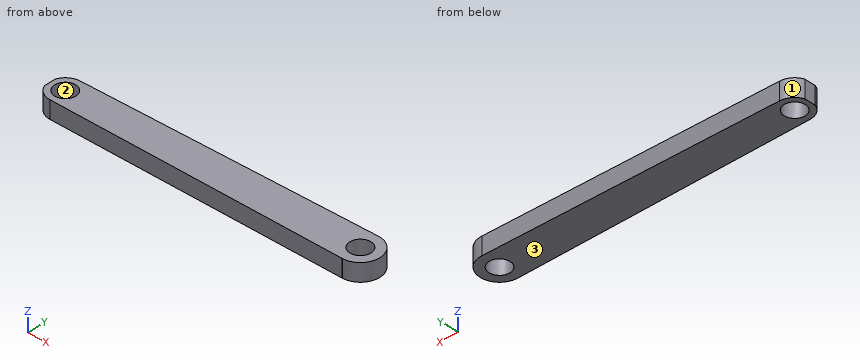
from build123d import *

# Parameters (mm, degrees)
SZKIC1_R                    = 4.635188213
SZKIC1_R_2                  = 3.000000079
SZKIC1_R_3                  = 5.522620658
DODANIE_WYCI_GNI_CIE1_DEPTH = 5
SZKIC2_W                    = 1.618528634
SZKIC2_H                    = 7.505645785
SZKIC2_W_2                  = 0.651830256
SZKIC2_H_2                  = 5.051684483
WYTNIJ_WYCI_GNI_CIE3_DEPTH  = 6


with BuildPart() as part:
    # Szkic1 → Dodanie-wyciągnięcie1 (new body)
    with BuildSketch(Plane.XY):
        with BuildLine():
            Line((0, -4.635188213), (83.645408354, -5.521381009))
            ThreePointArc((83.645408354, -5.521381009), (78.239794892, 0), (83.645408354, 5.521381009))
            Line((83.645408354, 5.521381009), (0, 4.635188213))
            ThreePointArc((0, 4.635188213), (3.277573017, 3.277573017), (4.635188213, 0))
            ThreePointArc((4.635188213, 0), (3.277573017, -3.277573017), (0, -4.635188213))
        make_face()
        Circle(SZKIC1_R)
        Circle(SZKIC1_R_2, mode=Mode.SUBTRACT)
        with BuildLine():
            ThreePointArc((0, 4.635188213), (-4.635188213, 0), (0, -4.635188213))
            ThreePointArc((0, -4.635188213), (3.277573017, -3.277573017), (4.635188213, 0))
            ThreePointArc((4.635188213, 0), (3.277573017, 3.277573017), (0, 4.635188213))
        make_face()
        Circle(SZKIC1_R_2, mode=Mode.SUBTRACT)
        with BuildLine():
            ThreePointArc((83.645408354, -5.521381009), (83.703908669, -5.522310737), (83.76241555, -5.522620658))
            Line((83.76241555, -5.522620658), (83.645408354, -5.521381009))
        make_face()
        with Locations((83.76241555, 0)):
            Circle(SZKIC1_R_3)
        with Locations((83.76241555, 0)):
            Circle(SZKIC1_R_2, mode=Mode.SUBTRACT)
        with BuildLine():
            ThreePointArc((83.76241555, 5.522620658), (83.703908669, 5.522310737), (83.645408354, 5.521381009))
            Line((83.645408354, 5.521381009), (83.76241555, 5.522620658))
        make_face()
    extrude(amount=DODANIE_WYCI_GNI_CIE1_DEPTH)

    # Szkic2 → Wytnij-wyciągnięcie3 (cut, through all)
    with BuildSketch(Plane.XY):
        with Locations((193.638606269, 0.381285041)):
            Rectangle(SZKIC2_W, SZKIC2_H)
        with Locations((-4.682734605, -0.038745932)):
            Rectangle(SZKIC2_W_2, SZKIC2_H_2)
    extrude(amount=WYTNIJ_WYCI_GNI_CIE3_DEPTH, mode=Mode.SUBTRACT)


solid = part.part
CAD build for the part. Positions are in the model's coordinates, mm. Face numbers are marked on the shaded views. Round coordinates to 2 decimals unless told otherwise and drop trailing zeros. Write each loop counter-clockwise with the first axis right and the second up, starting at its lowest first coordinate (ties: lowest second). Pieces come first, ordered by that corner, then holes. Notation, with made-up numbers: M 33,35.25 L 39,35.25 A13 ccw 39,55.25 Z; hole C -40,6 d7. An arc over 180 degrees is marked long. Put each result on its own line as item: value. Start each with the question number.
1) Pin check, flat tips, straight feed: pin 1 Ø1 at (x, z) = (19.5, 1.5) entering from -Y; pin 2 Ø5 at (x, y) = (0, 0) entering from -Z. Stop position of each tip, or through.
2) Saw through at B-B, the plane y = 0. Write the cut outline in (x, z), and give its area (3 significant figures).
3) Pull direction Y, two halves, no side cores. Call the marked faces 1, 2 and 3: pulls with the +Y half, pulls with the -Y half, needs draft (parallel to the pull), parting line crosses it, or undercut.
4) Saw through at A-A, the plane z = 3. Write the cut outline in (x, y), and give its area (3 significant figures).
5) Saw through at C-C, the plane x = 52.5. Write the cut outline in (y, z).
6) Drill centre lines: probe 1 along X at (y, z) = (-1.25, 2.5); probe 2 along X at (y, z) = (1.5, 2.7); probe 3 along Y at (x, z) = (0, 3.7). Where is each one in solid material? Low to high. Write a range as [from, to].
7) Saw through at D-D, the plane x = 29.5. Write the cut outline in (y, z), and give its area (3 significant figures).
Resolved:
1. pin 1: y = -4.85
1. pin 2: through
2. outline: M -4.36,0 L -3,0 L -3,5 L -4.36,5 Z; M 3,0 L 80.76,0 L 80.76,5 L 3,5 Z; M 86.76,0 L 89.29,0 L 89.29,5 L 86.76,5 Z
2. area: 408 mm²
3. face 1: pulls with the +Y half
3. face 2: undercut
3. face 3: needs draft
4. outline: M -4.36,-1.58 A4.64 ccw 0,-4.64 L 83.65,-5.52 A5.52 ccw long 83.65,5.52 L 0,4.64 A4.64 ccw -4.36,1.58 Z; hole C 0,0 d6; hole C 83.76,0 d6
4. area: 875 mm²
5. outline: M -5.19,0 L 5.19,0 L 5.19,5 L -5.19,5 Z
6. probe 1: [-4.36, -2.73], [2.73, 81.04], [86.49, 89.14]
6. probe 2: [-4.36, -2.6], [2.6, 81.16], [86.36, 89.08]
6. probe 3: [-4.64, -3], [3, 4.64]
7. outline: M -4.95,0 L 4.95,0 L 4.95,5 L -4.95,5 Z
7. area: 49.5 mm²
